from build123d import *

# Parameters (mm, degrees)
BOSS_EXTRUDE1_DEPTH    = 48
M2_5_CLEARANCE_HOLE2_D = 2.7
M2_5_CLEARANCE_HOLE3_D = 2.7


with BuildPart() as part:
    # Sketch3 → Boss-Extrude1 (new body)
    with BuildSketch(Plane.XY.offset(10)):
        Polygon((-8, 13), (-3.5, 13), (-3.5, 16), (-5, 16), (-5, 18.5), (5, 18.5), (5, 16), (3.5, 16), (3.5, 13), (14.25, 13), (14.25, 80.88), (7, 80.88), (7, 23), (-8, 23), align=None)
    extrude(amount=-BOSS_EXTRUDE1_DEPTH)

    # M2.5 Clearance Hole2 (through all)
    with Locations(Plane(origin=(0, 23, 0), x_dir=(1, 0, 0), z_dir=(0, 1, 0))):
        with Locations((0, 14)):
            Hole(M2_5_CLEARANCE_HOLE2_D / 2)

    # M2.5 Clearance Hole3 (through all)
    with Locations(Plane.ZY.offset(-7)):
        with Locations((-14, 70.44), (-14, 33.44)):
            Hole(M2_5_CLEARANCE_HOLE3_D / 2)


solid = part.part
Here's how the part is built. I have some questions about the finished solid (model axes, mm). A direction names the side the tool comes from. Coordinates: 2 decimals unless noted, no trailing zeros. Loops run counter-clockwise (first coordinate to the right, second up) from the corner with the lowest first, then second, coordinate; pieces in that order, holes last. Notation, with made-up numbers: (-36.5, -8) -> (14.5, -8) arc R25 cw to (14.5, 11) -> close; hole circle Ø8 at (18.25, 66). An arc over 180 degrees is marked (long way). Use one line per item in the form item = value. Start each with the question number.
(1) Will these pins go through, and if not, where does the flat tip stop? pin 1 (8 mm diameter, centred on y = 66, z = -22.5, fed in from -X); pin 2 (1.2 mm diameter, centred on x = 4, z = -19.5, fed in from +Y); pin 3 (4.5 mm diameter, centred on x = 0, z = -14, fed in from -Y).
(2) If we section it at B-B (x = 0): Please give me the cut outline in (y, z).
(3) If we section it at C-C (z = -14): Please give me the cut outline in (x, y).
(4) Please list where these lines run through material, in increasing order: line 1 along Z through (x, y) = (0, 21.3); line 2 along Y through (x, z) = (11.75, -14); line 3 along Y through (x, z) = (6.5, -25).
(5) We'd pull the mould along Z, two halves only. Please class faces 5 (the face through (-8, 18, -14)), 6 (the face through (10, 42, 10)), 7 (the face through (0.176, 20.719, -15.339)): pulls with the +Z half, pulls with the -Z half, needs draft (parallel to the pull), parting line crosses it, or undercut.
(6) If we section it at D-D (y = 46): Please give me the cut outline in (x, z), then the cut area to 3 significant figures.
(7) If we section it at A-A (y = 70.44): Please give me the cut outline in (x, z), then the cut area to 3 significant figures.
(8) On a 3-axis mill with a long thin cutter (end or side, diameter ignored), from which of +Z, -Z, +X, -X, +Y, -Y can I reach the whole of each face in a straight line? I mean faces 1 (the face through (-4, 16, -14)), 2 (the face through (-2, 23, -14)), 3 (the face through (10.68, 32.12, -13.71)), 4 (the face through (-3.5, 14, -14)). Say none if no direction works.
Verdict:
q1.pin_1 = 7
q1.pin_2 = 23
q1.pin_3 = 18.5
q2.outline = (18.5, -38) -> (23, -38) -> (23, -15.35) -> (18.5, -15.35) -> close; (18.5, -12.65) -> (23, -12.65) -> (23, 10) -> (18.5, 10) -> close
q3.outline = (-8, 13) -> (-3.5, 13) -> (-3.5, 16) -> (-5, 16) -> (-5, 18.5) -> (-1.35, 18.5) -> (-1.35, 23) -> (-8, 23) -> close; (1.35, 18.5) -> (5, 18.5) -> (5, 16) -> (3.5, 16) -> (3.5, 13) -> (14.25, 13) -> (14.25, 32.09) -> (7, 32.09) -> (7, 23) -> (1.35, 23) -> close; (7, 34.79) -> (14.25, 34.79) -> (14.25, 69.09) -> (7, 69.09) -> close; (7, 71.79) -> (14.25, 71.79) -> (14.25, 80.88) -> (7, 80.88) -> close
q4.line_1 = -38 to -15.35, -12.65 to 10
q4.line_2 = 13 to 32.09, 34.79 to 69.09, 71.79 to 80.88
q4.line_3 = 13 to 23
q5.face_5 = needs draft
q5.face_6 = pulls with the +Z half
q5.face_7 = undercut
q6.outline = (7, -38) -> (14.25, -38) -> (14.25, 10) -> (7, 10) -> close
q6.area = 348 mm²
q7.outline = (7, -38) -> (14.25, -38) -> (14.25, -15.35) -> (7, -15.35) -> close; (7, -12.65) -> (14.25, -12.65) -> (14.25, 10) -> (7, 10) -> close
q7.area = 328 mm²
q8.face_1 = +Z, -Z
q8.face_2 = +Z, -Z, -X, +Y
q8.face_3 = +X, -X
q8.face_4 = +Z, -Z, -Y
